Could you check a few things on this model? Use its own coordinates, in mm. A direction names the side the tool comes from. Round coordinates to 2 decimals unless told otherwise and drop trailing zeros. Order: outer loops, then holes, each group sorted by start corner. A loop starts at its lowest first (then second) coordinate and runs counter-clockwise, first axis right, second up. Notation, with made-up numbers: (75, 80) - (122, 80) arc R23 ccw to (122, 90) - close; hole circle Ø1 at (-18.75, -0.75). An arc over 180 degrees is marked (long way). Use one line per item in the form item = value.
from build123d import *

# Parameters (mm, degrees)
F1_DEPTH = 18
F2_R     = 5
F3_R     = 2.5


with BuildPart() as f1:
    # F0 (on Top) → F1 (new body)
    with BuildSketch(Plane.XY):
        with BuildLine():
            Line((0, 70), (0, 0))
            Line((0, 0), (166, 0))
            Line((166, 0), (166, 47))
            ThreePointArc((166, 47), (163.87868, 52.12132), (169, 50))
            Line((169, 50), (181, 50))
            ThreePointArc((181, 50), (184, 53), (187, 50))
            ThreePointArc((187, 50), (186.12132, 47.87868), (184, 47))
            Line((184, 47), (184, 0))
            Line((184, 0), (200, 0))
            Line((200, 0), (200, 70))
            Line((200, 70), (34, 70))
            Line((34, 70), (34, 23))
            ThreePointArc((34, 23), (36.12132, 22.12132), (37, 20))
            ThreePointArc((37, 20), (34, 17), (31, 20))
            Line((31, 20), (19, 20))
            ThreePointArc((19, 20), (13.87868, 17.87868), (16, 23))
            Line((16, 23), (16, 70))
            Line((16, 70), (0, 70))
        make_face()
    extrude(amount=F1_DEPTH)

    # F2
    f2_edges = [f1.edges().sort_by_distance(p)[0] for p in [
        (0, 0, 9),
        (200, 70, 9),
        (200, 0, 9),
        (0, 70, 9),
    ]]
    fillet(f2_edges, radius=F2_R)

    # F3
    f3_edges = [f1.edges().sort_by_distance(p)[0] for p in [
        (85.5, 0, 18),
        (85.5, 0, 0),
        (114.5, 70, 18),
        (200, 35, 0),
    ]]
    fillet(f3_edges, radius=F3_R)


solid = f1.part
Item 1: For faces 4 (the face through (175, 50, 9)), 5 (the face through (34, 47, 9)), 6 (the face through (84, 0, 9)), which set-ups out of +Z, -Z, +X, -X, +Y, -Y let a thin tool reach every point of the face, with its end or its side?
Found:
face_4 = +Z, -Z, -Y
face_5 = +Z, -Z, +Y
face_6 = +Z, -Z, +X, -X, -Y
Item 2: I need wall thicknesses on L1, parallel to X at y = 32, z = 9.25; L2, parallel to X at y = 13, z = 6.5; L3, parallel to X at y = 22, z = 8.25. Which ranges of each line are inside material? Lowest first, please.
Found:
L1 = 0 to 16, 34 to 166, 184 to 200
L2 = 0 to 166, 184 to 200
L3 = 0 to 13.76, 36.24 to 166, 184 to 200
Item 3: Imagine slicing it at D-D on x = 22. Please give me the cut outline in (y, z), plus the area to 3 significant figures.
Found:
outline = (0, 2.5) arc R2.5 ccw to (2.5, 0) - (20, 0) - (20, 18) - (2.5, 18) arc R2.5 ccw to (0, 15.5) - close
area = 357 mm2
Item 4: If we mould it in two halves opening along Y, with no side actions, what happens to faces 1 (the face through (11, 70, 9)), 2 (the face through (1, 2, 9)), 3 (the face through (163.81, 52.05, 8.87))? For each: released by +Y, released by -Y, zero draft, split by the parting line, or undercut.
Found:
face_1 = released by +Y
face_2 = released by -Y
face_3 = undercut
Item 5: Will these pins go through, and if not, where does the flat tip stop? P1, Ø6, axis at x = 27, z = 5, coming from the +Y side; P2, Ø9.5, axis at x = 176.5, z = 7.5, coming from the -Y side.
Found:
P1 = 20
P2 = 50
Item 6: Imagine slicing it at A-A on y = 58.5. Please give me the cut outline in (x, z).
Found:
outline = (0, 2.5) arc R2.5 ccw to (2.5, 0) - (16, 0) - (16, 18) - (2.5, 18) arc R2.5 ccw to (0, 15.5) - close; (34, 0) - (197.5, 0) arc R2.5 ccw to (200, 2.5) - (200, 15.5) arc R2.5 ccw to (197.5, 18) - (34, 18) - close
Item 7: Imagine slicing it at C-C on z = 9.5. Please give me the cut outline in (x, y).
Found:
outline = (0, 5) arc R5 ccw to (5, 0) - (166, 0) - (166, 47) arc R3 cw (long way) to (169, 50) - (181, 50) arc R3 cw to (187, 50) arc R3 cw to (184, 47) - (184, 0) - (195, 0) arc R5 ccw to (200, 5) - (200, 65) arc R5 ccw to (195, 70) - (34, 70) - (34, 23) arc R3 cw to (37, 20) arc R3 cw to (31, 20) - (19, 20) arc R3 cw (long way) to (16, 23) - (16, 70) - (5, 70) arc R5 ccw to (0, 65) - close
Item 8: Imagine slicing it at B-B on y = 33.5. Please give me the cut outline in (x, z), plus the area to 3 significant figures.
Found:
outline = (0, 2.5) arc R2.5 ccw to (2.5, 0) - (16, 0) - (16, 18) - (2.5, 18) arc R2.5 ccw to (0, 15.5) - close; (34, 0) - (166, 0) - (166, 18) - (34, 18) - close; (184, 0) - (197.5, 0) arc R2.5 ccw to (200, 2.5) - (200, 15.5) arc R2.5 ccw to (197.5, 18) - (184, 18) - close
area = 2,950 mm2
